Can you work these out from the drawing? Everything is in mm from the part's minimum corner. Coordinates: 2 decimals unless noted, no trailing zeros. Order: outer loops, then holes, each group sorted by start corner. A loop starts at its lowest first (then second) coordinate and runs counter-clockwise, first axis right, second up. Notation, with made-up numbers: (55.25, 31) -> (107.25, 31) arc R22 cw to (107.25, 61) -> close; hole circle Ø9 at (76, -10). An arc over 180 degrees is marked (long way). Answer in a Markdown table with one row per item.
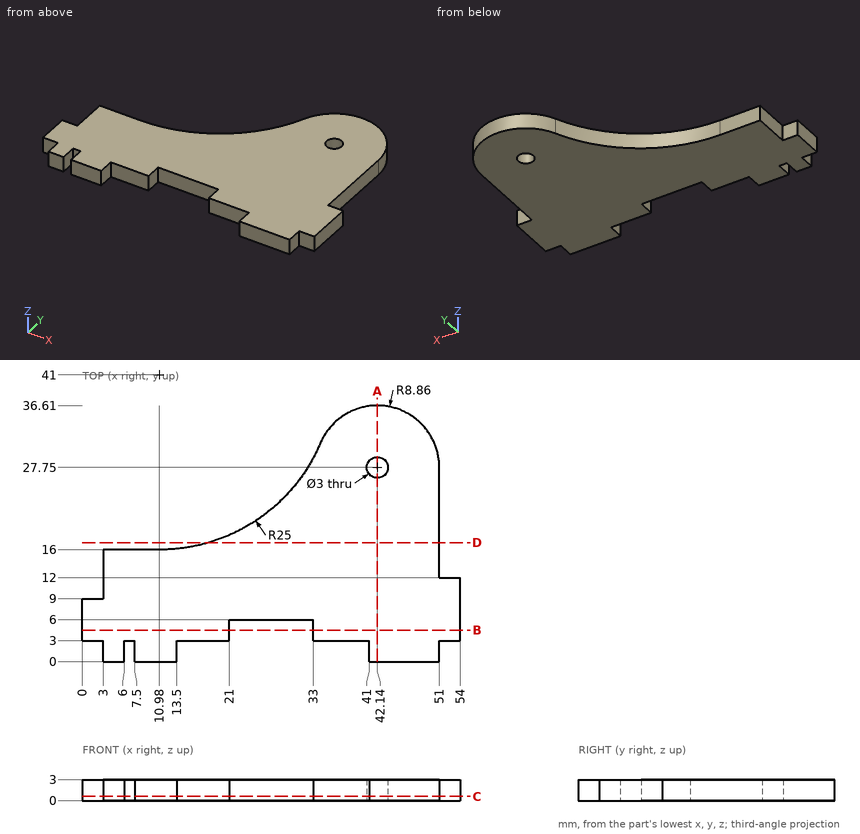
(1) Suppose I cut it at B-B (y = 4.5). Please give me the cut outline in (x, z), and give its area (3 significant figures).
Response values:
| item | result |
|---|---|
| outline | (0, 0) -> (21, 0) -> (21, 3) -> (0, 3) -> close; (33, 0) -> (54, 0) -> (54, 3) -> (33, 3) -> close |
| area | 126 mm2 |
(2) Suppose I cut it at A-A (x = 42.14). Please give me the cut outline in (y, z).
Response values:
| item | result |
|---|---|
| outline | (0, 0) -> (26.25, 0) -> (26.25, 3) -> (0, 3) -> close; (29.25, 0) -> (36.61, 0) -> (36.61, 3) -> (29.25, 3) -> close |
(3) Will these pins go through, and if not, where does the flat tip stop? pin 1 Ø0.9 at (x, z) = (52, 2) entering from -Y; pin 2 Ø1.5 at (x, z) = (29, 1) entering from -Y; pin 3 Ø1 at (x, z) = (48, 1.5) entering from -Y; pin 4 Ø0.9 at (y, z) = (2, 2) entering from +X.
Response values:
| item | result |
|---|---|
| pin 1 | y = 3 |
| pin 2 | y = 6 |
| pin 3 | y = 0 |
| pin 4 | x = 51 |
(4) Suppose I cut it at D-D (y = 17). Please give me the cut outline in (x, z).
Response values:
| item | result |
|---|---|
| outline | (17.98, 0) -> (51, 0) -> (51, 3) -> (17.98, 3) -> close |
(5) I need wall thicknesses on line 1 (Y direction, x = 42.14, z = 1.35); line 2 (X direction, y = 2.5, z = 0.6); line 3 (X direction, y = 26.5, z = 2.45) (1 decimal). Which ranges of each line are inside material? Lowest first, please. Write a range as [from, to].
Response values:
| item | result |
|---|---|
| line 1 | [0, 26.25], [29.25, 36.61] |
| line 2 | [3, 6], [7.5, 13.5], [41, 51] |
| line 3 | [31.3, 41.3], [43, 51] |
(6) Suppose I cut it at C-C (z = 0.6). Please give me the cut outline in (x, y), and give its area (3 significant figures).
Response values:
| item | result |
|---|---|
| outline | (0, 3) -> (3, 3) -> (3, 0) -> (6, 0) -> (6, 3) -> (7.5, 3) -> (7.5, 0) -> (13.5, 0) -> (13.5, 3) -> (21, 3) -> (21, 6) -> (33, 6) -> (33, 3) -> (41, 3) -> (41, 0) -> (51, 0) -> (51, 3) -> (54, 3) -> (54, 12) -> (51, 12) -> (51, 27.75) arc R8.86 ccw to (33.99, 31.22) arc R25 cw to (10.98, 16) -> (3, 16) -> (3, 9) -> (0, 9) -> close; hole circle Ø3 at (42.14, 27.75) |
| area | 1,100 mm2 |
